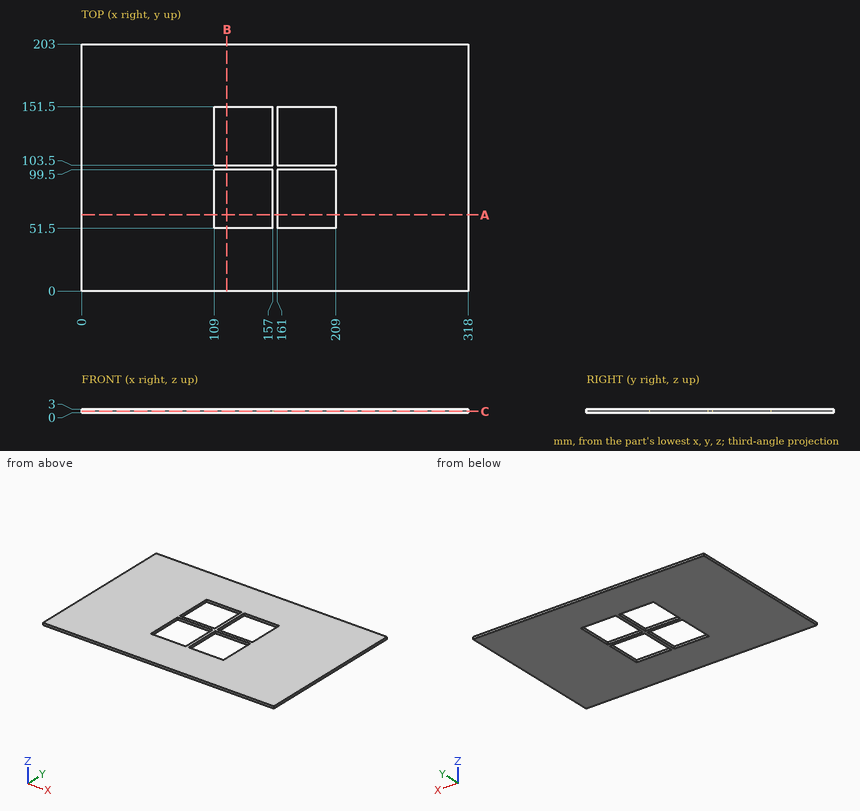
Check sheet for the drawn part. Datum: minimum x, y, z corner. Units: mm. Round coordinates to 2 decimals unless told otherwise and drop trailing zeros. Order: outer loops, then holes, each group sorted by start corner. A loop starts at its lowest first (then second) coordinate and runs counter-clockwise, first axis right, second up.
(1) Cross-section at A-A, the plane y = 62.5. Enter the section's corners in (x, z), and give its area (3 significant figures).
(2) Cross-section at C-C, the plane z = 1.15. Enter the section's corners in (x, y), and give its area (3 significant figures).
(3) Cross-section at B-B, the plane x = 119.5. Enter the section's corners in (y, z).
(4) Scan lines: probe 1 along Y at (x, z) = (187.5, 0.6); probe 2 along X at (y, z) = (69, 2.8). Record each from-to range of solid material in increasing order.
Check sheet entries:
1. outline: (0, 0) - (109, 0) - (109, 3) - (0, 3) - close; (157, 0) - (161, 0) - (161, 3) - (157, 3) - close; (209, 0) - (318, 0) - (318, 3) - (209, 3) - close
1. area: 666 mm2
2. outline: (0, 0) - (318, 0) - (318, 203) - (0, 203) - close; hole (109, 51.5) - (157, 51.5) - (157, 99.5) - (109, 99.5) - close; hole (109, 103.5) - (157, 103.5) - (157, 151.5) - (109, 151.5) - close; hole (161, 51.5) - (209, 51.5) - (209, 99.5) - (161, 99.5) - close; hole (161, 103.5) - (209, 103.5) - (209, 151.5) - (161, 151.5) - close
2. area: 55,300 mm2
3. outline: (0, 0) - (51.5, 0) - (51.5, 3) - (0, 3) - close; (99.5, 0) - (103.5, 0) - (103.5, 3) - (99.5, 3) - close; (151.5, 0) - (203, 0) - (203, 3) - (151.5, 3) - close
4. probe 1: y = 0 to 51.5, 99.5 to 103.5, 151.5 to 203
4. probe 2: x = 0 to 109, 157 to 161, 209 to 318
